Build history of the part. All positions in model axes, mm. A direction names the side the tool comes from. Give positions to 0.01 mm unless a question says otherwise; leave off trailing zeros. Order: outer loops, then holes, each group sorted by start corner. A loop starts at its lowest first (then second) coordinate and runs counter-clockwise, first axis right, second up. Notation, with made-up numbers: (19.25, 4.25) -> (54.25, 4.25) arc R13 cw to (54.25, 17.25) -> close; hole circle Ø9 at (52, 75.25). An arc over 180 degrees is marked (long way). Use a Markdown table: item, result. Add a question column.
```python
from build123d import *

# Parameters (mm, degrees)
F0_R     = 2.4986506911
F1_DEPTH = 3.0734
F2_R     = 8.8528062314
F2_R_2   = 7.6336843155
F2_R_3   = 6.679620884
F2_R_4   = 4.5453115006
F2_R_5   = 0.5062861641
F3_DEPTH = 0.254


with BuildPart() as f1:
    # F0 (on Top) → F1 (new body)
    with BuildSketch(Plane.XY):
        with BuildLine():
            Line((-44.45, 88.9), (-44.45, 0))
            ThreePointArc((-44.45, 0), (0, -44.45), (44.45, 0))
            Line((44.45, 0), (44.45, 88.9))
            Line((44.45, 88.9), (-44.45, 88.9))
        make_face()
        with Locations((0, 82.8513503075)):
            Circle(F0_R, mode=Mode.SUBTRACT)
    extrude(amount=F1_DEPTH)

    # F2 (on face) → F3 (join)
    with BuildSketch(Plane.XY.offset(3.0734)):
        with Locations((0, 70.3227519989)):
            Circle(F2_R)
        with Locations((0, 70.3227519989)):
            Circle(F2_R_2, mode=Mode.SUBTRACT)
        with Locations((0, 70.3227519989)):
            Circle(F2_R_3)
        with Locations((0, 70.3227519989)):
            Circle(F2_R_4, mode=Mode.SUBTRACT)
        Polygon((-2.223612275, 71.8253105879), (-2.8203756083, 71.1344004551), (-2.4623177014, 69.4515183568), (-1.8788158195, 71.1344004551), align=None)
        Polygon((2.0716317148, 71.6240334723), (1.6487184912, 71.1344004551), (2.0716317148, 69.544352591), (2.6385103986, 71.1344004551), align=None)
        with Locations((0, 70.3227519989)):
            Circle(F2_R_5)
    extrude(amount=F3_DEPTH)


solid = f1.part
```
(1) Band-saw the part on C-C on y = -26. Give the cut face in (x, z).
(2) Mould opens along X. For faces 1 (the face through (1, 88.9, 2)), 2 (the face through (3, 64, 3.073)), 3 (the face through (-0.98, -44.44, 1.52)), 4 (the face through (-0.54, 80.41, 1.52)) say: released by +X, released by -X, zero draft, split by the parting line, or undercut.
(3) Band-saw the part on B-B on z = 0.55. Give the cut face in (x, y), plus the area to 3 significant figures.
(4) Band-saw the part on A-A on y = 39. Give the cut face in (x, z).
(5) Wall check: probe 1 along Y at (x, z) = (0, 3.2); probe 2 along Y at (x, z) = (0, 1.2); probe 3 along Z at (x, y) = (31.5, 6). Give the ranges that are in metal, low to high.
(6) Pin check, flat tips, straight feed: pin 1 Ø10 at (x, y) = (1, 69.5) entering from +Z; pin 2 Ø6 at (x, y) = (7, -30) entering from +Z; pin 3 Ø4 at (x, y) = (0, 82.85) entering from +Z (3 decimals). Stop position of each tip, or through.
(7) Tool access for faces 5 (the face through (44.45, 44, 2)), 6 (the face through (0, 69, 3.073)): list every direction of +Z, -Z, +X, -X, +Y, -Y with a clear straight run to the whole face (end or side of a thin tool).
Response:
| question | item | result |
|---|---|---|
| 1 | outline | (-36.05, 0) -> (36.05, 0) -> (36.05, 3.07) -> (-36.05, 3.07) -> close |
| 2 | face 1 | zero draft |
| 2 | face 2 | undercut |
| 2 | face 3 | split by the parting line |
| 2 | face 4 | undercut |
| 3 | outline | (-44.45, 0) arc R44.45 ccw to (44.45, 0) -> (44.45, 88.9) -> (-44.45, 88.9) -> close; hole circle Ø5 at (0, 82.85) |
| 3 | area | 11,000 mm² |
| 4 | outline | (-44.45, 0) -> (44.45, 0) -> (44.45, 3.07) -> (-44.45, 3.07) -> close |
| 5 | probe 1 | y = 61.47 to 62.69, 63.64 to 65.78, 69.82 to 70.83, 74.87 to 77, 77.96 to 79.18 |
| 5 | probe 2 | y = -44.45 to 80.35, 85.35 to 88.9 |
| 5 | probe 3 | z = 0 to 3.07 |
| 6 | pin 1 | stops at z = 3.33 |
| 6 | pin 2 | stops at z = 3.07 |
| 6 | pin 3 | passes through |
| 7 | face 5 | +Z, -Z, +X, +Y, -Y |
| 7 | face 6 | +Z |
